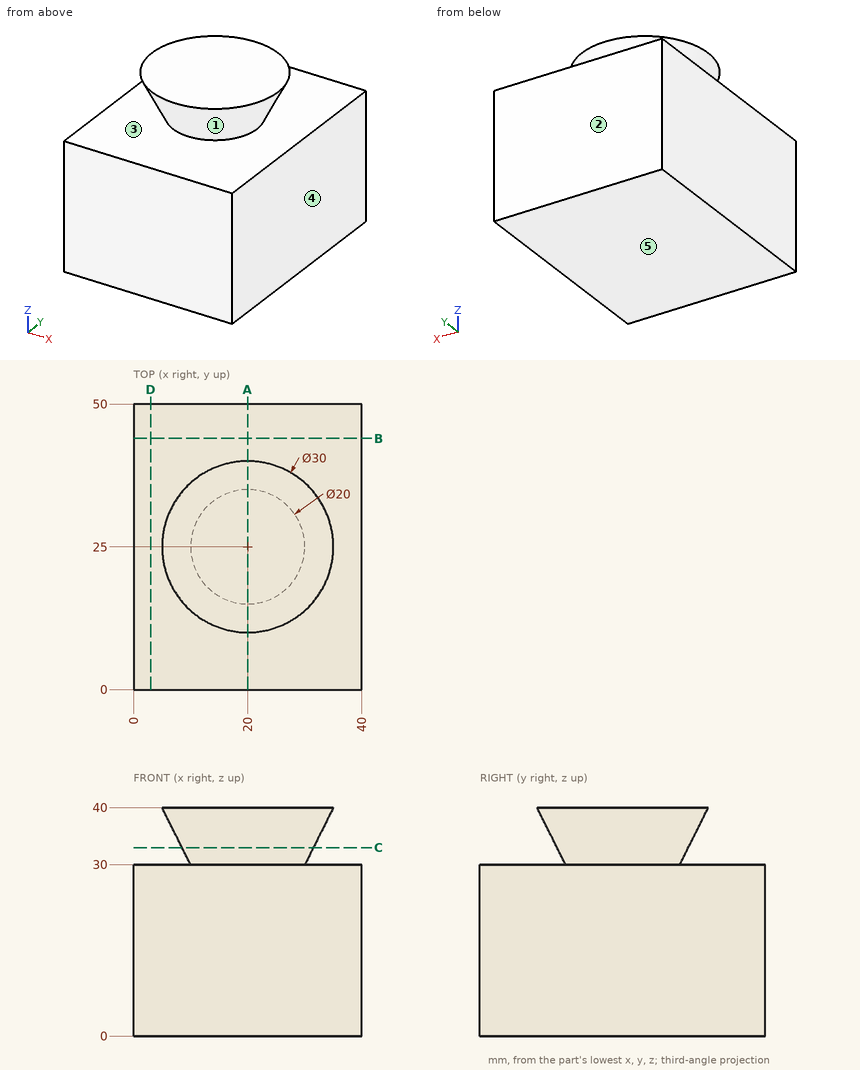
Could you check a few things on this drawing? It's one solid part, dimensions in mm from its lowest x, y, z. A direction names the side the tool comes from. Coordinates: 2 decimals unless noted, no trailing zeros. Order: outer loops, then holes, each group sorted by start corner. A loop starts at its lowest first (then second) coordinate and runs counter-clockwise, first axis right, second up. Notation, with made-up numbers: M 13.5,63.25 L 66.5,63.25 A19 cw 66.5,94.25 Z; hole C 5,-14 d9. An arc over 180 degrees is marked long. Use a Markdown table: item, result. Add a question column.
Q1. I want a section at C-C on z = 33. List the corners of the cut face in (x, y) for me, then the cut area to 3 significant figures.
Q2. We'd pull the mould along Z, two halves only. Please class the marked faces 3, 4 and 5: pulls with the +Z half, pulls with the -Z half, needs draft (parallel to the pull), parting line crosses it, or undercut.
Q3. Which directions (+Z, -Z, +X, -X, +Y, -Y) give clear straight access to the entire face, cutting with the end or side of a thin tool? Please do the marked faces 1 and 2.
Q4. I want a section at A-A on x = 20. List the corners of the cut face in (y, z) for me, then the cut area to 3 significant figures.
Q5. I want a section at B-B on y = 44. List the corners of the cut face in (x, z) for me, then the cut area to 3 significant figures.
Q6. I'm going to push flat-ended pins straight in: pin 1 (6 mm diameter, centred on y = 30.5, z = 34.5, fed in from +X); pin 2 (2 mm diameter, centred on x = 12, y = 10, fed in from +Z). Where does each tip first touch, or does it pass through?
Q7. If I drill on L1, parallel to Z at x = 15.5, y = 40.5; L2, parallel to Z at x = 28, y = 12.5; L3, parallel to Z at x = 26.5, y = 13, over which ranges is the centre line in solid material (lowest first)?
Q8. I want a section at D-D on x = 3. List the corners of the cut face in (y, z) for me, then the cut area to 3 significant figures.
Checked values:
| question | item | result |
|---|---|---|
| 1 | outline | C 20,25 d23 |
| 1 | area | 415 mm² |
| 2 | face 3 | undercut |
| 2 | face 4 | needs draft |
| 2 | face 5 | pulls with the -Z half |
| 3 | face 1 | none |
| 3 | face 2 | +Z, -Z, +X, -X, +Y |
| 4 | outline | M 0,0 L 50,0 L 50,30 L 35,30 L 40,40 L 10,40 L 15,30 L 0,30 Z |
| 4 | area | 1,750 mm² |
| 5 | outline | M 0,0 L 40,0 L 40,30 L 0,30 Z |
| 5 | area | 1,200 mm² |
| 6 | pin 1 | x = 32.95 |
| 6 | pin 2 | z = 30 |
| 7 | L1 | 0 to 30 |
| 7 | L2 | 0 to 30, 39.68 to 40 |
| 7 | L3 | 0 to 30, 37.29 to 40 |
| 8 | outline | M 0,0 L 50,0 L 50,30 L 0,30 Z |
| 8 | area | 1,500 mm² |
